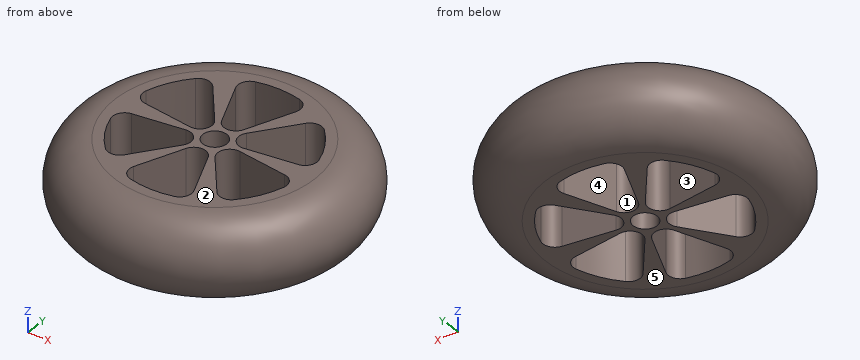
from build123d import *

# Parameters (mm, degrees)
SKETCH5_R           = 50
SKETCH5_R_2         = 6
BOSS_EXTRUDE2_DEPTH = 40
CUT_EXTRUDE1_DEPTH  = 41
CIRPATTERN1_COUNT   = 6


with BuildPart() as part:
    # Sketch5 → Boss-Extrude2 (new body)
    with BuildSketch(Plane.XY):
        Circle(SKETCH5_R)
        Circle(SKETCH5_R_2, mode=Mode.SUBTRACT)
    extrude(amount=BOSS_EXTRUDE2_DEPTH)

    # Sketch7 → Revolve3 (revolve)
    with BuildSketch(Plane(origin=(0, 0, 0), x_dir=(0, 0, -1), z_dir=(1, 0, 0))):
        with BuildLine():
            Line((-40, 50), (0, 50))
            ThreePointArc((0, 50), (-20, 70), (-40, 50))
        make_face()
    revolve(axis=Axis((0, 0, 40), (0, 0, -1)))

    # Sketch8 → Cut-Extrude1 (cut, through all)
    with BuildSketch(Plane.XY.offset(40)):
        with BuildLine():
            Line((5.543277195, 12.406847077), (15.113515228, 35.511445531))
            ThreePointArc((15.113515228, 35.511445531), (14.932932615, 40.498550922), (11.042582345, 43.624091683))
            ThreePointArc((11.042582345, 43.624091683), (0, 45), (-11.042582345, 43.624091683))
            ThreePointArc((-11.042582345, 43.624091683), (-14.932932615, 40.498550922), (-15.113515228, 35.511445531))
            Line((-15.113515228, 35.511445531), (-5.543277195, 12.406847077))
            ThreePointArc((-5.543277195, 12.406847077), (0, 8.702947672), (5.543277195, 12.406847077))
        make_face()
    cut_extrude1 = extrude(amount=-CUT_EXTRUDE1_DEPTH, mode=Mode.SUBTRACT)

    # CirPattern1: Cut-Extrude1 ×6 about axis
    cirpattern1_axis = Axis((0, 0, 0), (0, 0, 1))
    for i in range(1, CIRPATTERN1_COUNT):
        add(cut_extrude1.rotate(cirpattern1_axis, i * 360 / CIRPATTERN1_COUNT), mode=Mode.SUBTRACT)


solid = part.part
Geometry: final body of the model. Coordinates: model frame, mm. Face numbers are marked on the shaded views. A direction names the side the tool comes from. Coordinates: 2 decimals unless noted, no trailing zeros. Loops run counter-clockwise (first coordinate to the right, second up) from the corner with the lowest first, then second, coordinate; pieces in that order, holes last. Notation, with made-up numbers: (2, 53.5) - (46, 53.5) arc R31 cw to (46, 91.5) - close; hole circle Ø3 at (25, 12.5). An arc over 180 degrees is marked (long way). One line per question, with ' | ' between items. Start each with the question number.
(1) Ray query, L1, parallel to Y at x = 14, z = 4; L2, parallel to Y at x = 25, z = 24; L3, parallel to Y at x = 26.5, z = 8. Return the intervals inside material, ascending. Write a range as from..to.
(2) Cut plane B-B on z = 8. Count the separate pieces of the cut face and the enclosed holes in it, and give its area (3 significant figures).
(3) First-contact query: pin 1 (12 mm diameter, centred on y = -11, z = 34.5, fed in from -X); pin 2 (5 mm diameter, centred on y = -16.5, z = 12, fed in from -X); pin 3 (10 mm diameter, centred on y = 50, z = 7.5, fed in from +X). Flat tips, straight axial feed; report the tip coordinate or a pass-through.
(4) Draft query along Y for the marked faces 3, 4 and 5. Return one class per face: +Y half, -Y half, draft (parallel to the pull), parting line (faces both ways), or undercut.
(5) Reachability of the marked faces 1 and 2 from +Z, -Z, +X, -X, +Y, -Y: full face, straight path, thin tool, end or side. Return the list, or none.
(6) Cut plane A-A on x = 0. Output: boundary loops of the cut face in (y, z).
Here are the results:
1) L1: -60.4..-41.85, -32.82..-18.86, -1.47..1.47, 18.86..32.82, 41.85..60.4 | L2: -64.95..-32.41, -2.91..2.91, 32.41..64.95 | L3: -60.45..-33.01, -3.11..3.11, 33.01..60.45
2) separate pieces: 1 | enclosed holes: 7 | area: 8,980 mm²
3) pin 1: x = -67.35 | pin 2: x = -67.43 | pin 3: x = 49.54
4) face 3: undercut | face 4: undercut | face 5: draft
5) face 1: +Z, -Z | face 2: +Z, +X, -X, +Y, -Y
6) outline: (-50, 0) - (-45, 0) - (-45, 40) - (-50, 40) arc R20 ccw to start; (-8.7, 0) - (-6, 0) - (-6, 40) - (-8.7, 40) - close; (6, 0) - (8.7, 0) - (8.7, 40) - (6, 40) - close; (45, 0) - (50, 0) arc R20 ccw to (50, 40) - (45, 40) - close
